The figure shows three views and two pictorial views of one solid part (mm, origin at its lowest corner). Answer the questions. A direction names the side the tool comes from. Coordinates: 2 decimals unless noted, no trailing zeros. Order: outer loops, then holes, each group sorted by start corner. A loop starts at its lowest first (then second) coordinate and runs counter-clockwise, first axis right, second up. Notation, with made-up numbers: (88, 76.25) -> (101, 76.25) arc R30 cw to (101, 111.25) -> close; hole circle Ø9 at (67.25, -9). An arc over 180 degrees is marked (long way). Write item = value, one per line. Start each with the question number.
Q1. Which of the six approach directions +Z, -Z, +X, -X, +Y, -Y give full straight-line access (tool end or side, diameter ignored) to the marked faces 1, 2 and 3?
Q2. The part is cut by section A-A, the plane z = 2. Count the separate pieces of the cut face and the enclosed holes in it, plus the area to 3 significant figures.
Q3. Straight lines are drawn through the part: L1, parallel to X at y = 3.45, z = 1.5; L2, parallel to Y at x = 4.91, z = 5.5 (1 decimal); L3, parallel to Z at x = 16.75, y = 2.9. For each, find the intervals that lie inside material, in ascending order. Write a range as from..to.
Q4. For a pull along X with two mould halves and no side action, classify the marked faces 4, 5 and 6 as +X half, -X half, draft (parallel to the pull), parting line (faces both ways), or undercut.
Q5. The part is cut by section D-D, the plane z = 10. Determine the outline of the cut face in (x, y) (3 decimals), plus the area to 3 significant figures.
Q6. Flat-ended cylindrical pins translate along their axes: pin 1 (1.9 mm diameter, centred on x = 4.91, y = 2.5, fed in from +Z); pin 2 (2.5 mm diameter, centred on x = 12.875, y = 2.5, fed in from +Z); pin 3 (4 mm diameter, centred on x = 5, z = 5, fed in from +Y) (3 decimals). Find the tip coordinate at first contact, or state that the pin passes through.
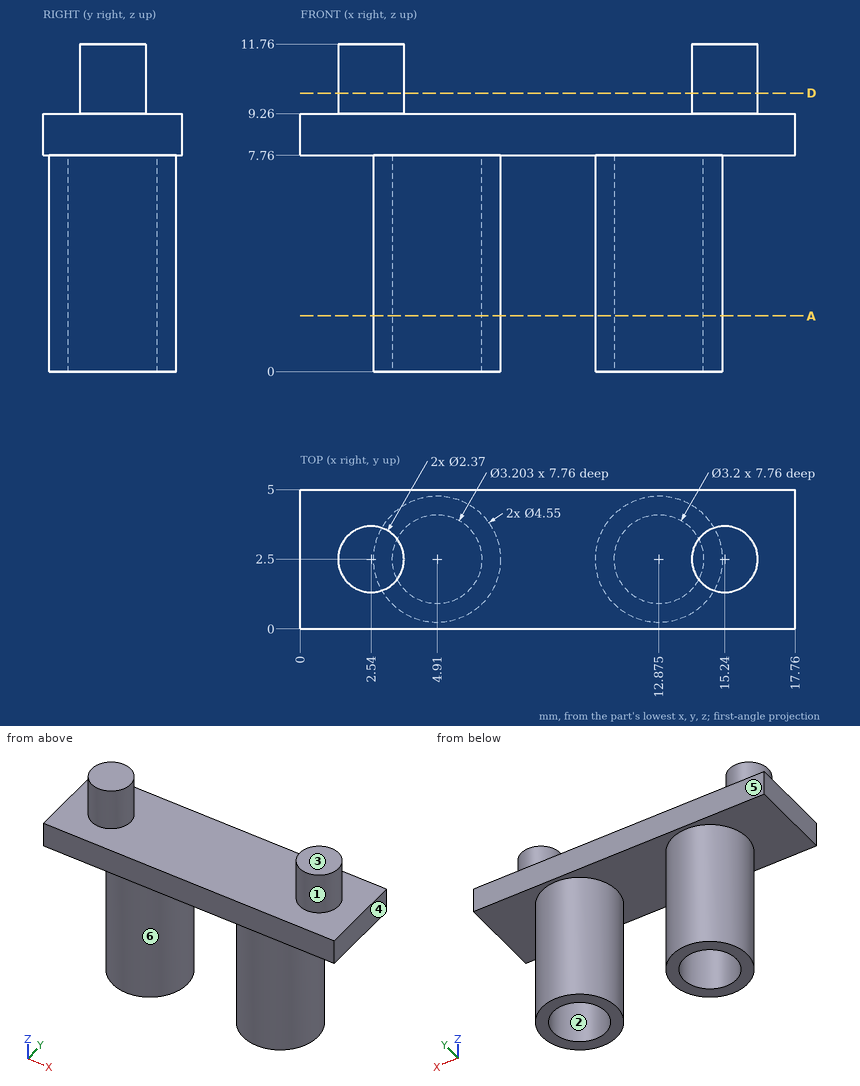
Model answer:
q1.face_1 = +Z
q1.face_2 = -Z
q1.face_3 = +Z, +X, -X, +Y, -Y
q2.separate_pieces = 2
q2.enclosed_holes = 2
q2.area = 16.4 mm2
q3.L1 = 2.84..3.62, 6.2..6.98, 10.81..11.59, 14.16..14.94
q3.L2 = 0.2..0.9, 4.1..4.8
q3.L3 = 7.76..9.26
q4.face_4 = +X half
q4.face_5 = draft
q4.face_6 = undercut
q5.outline = circle Ø2.37 at (2.54, 2.5); circle Ø2.37 at (15.24, 2.5)
q5.area = 8.82 mm2
q6.pin_1 = 9.26
q6.pin_2 = 11.76
q6.pin_3 = 4.775
